```python
from build123d import *

# Parameters (mm, degrees)
F0_R     = 10.978044
F0_W     = 4.940685
F0_H     = 7.991237
F0_R_2   = 1.481086
F0_W_2   = 4.940115
F0_H_2   = 7.966079
F0_W_3   = 5.002896
F0_H_3   = 8.001204
F0_R_3   = 1.470755
F0_W_4   = 4.997425
F0_H_4   = 7.974718
F1_DEPTH = 5.0038


with BuildPart() as f1:
    # F0 (on Front) → F1 (new body)
    with BuildSketch(Plane.XZ):
        Polygon((29.282646, 29.627208), (-30.758047, 29.627208), (-30.758047, -12.548319), (-22.847719, -12.548319), (-22.847719, -63.122556), (21.501994, -63.122556), (21.501994, -12.548319), (29.282646, -12.548319), align=None)
        with BuildLine():
            ThreePointArc((-15.586378, -40.243281), (-17.742358, -40.254847), (-17.64737, -38.100929))
            Line((-17.64737, -38.100929), (-14.625554, -35.052073))
            ThreePointArc((-14.625554, -35.052073), (-12.57034, -35.03634), (-12.541453, -37.091411))
            Line((-12.541453, -37.091411), (-15.586378, -40.243281))
        make_face(mode=Mode.SUBTRACT)
        with BuildLine():
            ThreePointArc((16.426139, -38.233279), (16.534977, -40.292482), (14.478289, -40.441467))
            Line((14.478289, -40.441467), (11.236794, -37.068415))
            ThreePointArc((11.236794, -37.068415), (11.464462, -35.022049), (13.520983, -35.12287))
            ThreePointArc((13.520983, -35.12287), (13.537568, -35.140344), (13.55387, -35.158081))
            Line((13.55387, -35.158081), (16.426139, -38.233279))
        make_face(mode=Mode.SUBTRACT)
        with Locations((-0.654383, -23.181881)):
            Circle(F0_R, mode=Mode.SUBTRACT)
        with Locations((-25.189546, -3.442893)):
            Rectangle(F0_W, F0_H, mode=Mode.SUBTRACT)
        with BuildLine():
            ThreePointArc((-17.563489, -8.410167), (-17.594804, -6.240676), (-15.426944, -6.330432))
            Line((-15.426944, -6.330432), (-12.764063, -8.947979))
            ThreePointArc((-12.764063, -8.947979), (-12.531586, -11.12918), (-14.723433, -11.21573))
            Line((-14.723433, -11.21573), (-17.563489, -8.410167))
        make_face(mode=Mode.SUBTRACT)
        with Locations((-25.166028, 8.524365)):
            Circle(F0_R_2, mode=Mode.SUBTRACT)
        with Locations((-25.189262, 20.554467)):
            Rectangle(F0_W_2, F0_H_2, mode=Mode.SUBTRACT)
        with BuildLine():
            ThreePointArc((14.199827, -6.306034), (16.317638, -6.34597), (16.353841, -8.463848))
            Line((16.353841, -8.463848), (13.079717, -11.405483))
            ThreePointArc((13.079717, -11.405483), (10.953875, -11.342186), (11.064754, -9.218293))
            Line((11.064754, -9.218293), (14.199827, -6.306034))
        make_face(mode=Mode.SUBTRACT)
        with Locations((23.799085, -3.43791)):
            Rectangle(F0_W_3, F0_H_3, mode=Mode.SUBTRACT)
        with Locations((23.838598, 8.52569)):
            Circle(F0_R_3, mode=Mode.SUBTRACT)
        with Locations((23.80182, 20.558786)):
            Rectangle(F0_W_4, F0_H_4, mode=Mode.SUBTRACT)
    extrude(amount=F1_DEPTH)


solid = f1.part
```
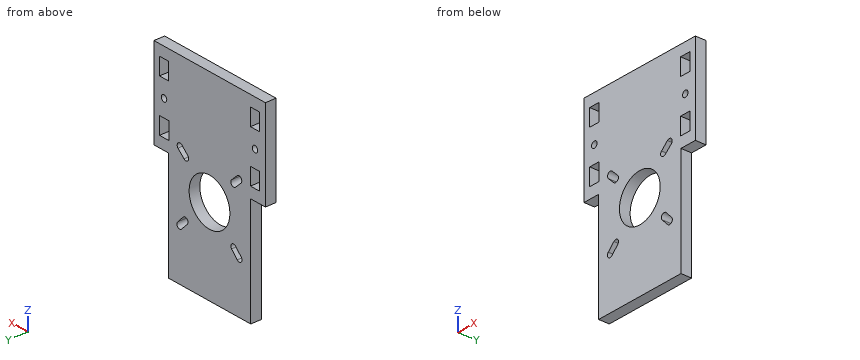
Here's how the part is built. I have some questions about the finished solid (model axes, mm). Give positions to 0.01 mm unless a question says otherwise; leave off trailing zeros. Order: outer loops, then holes, each group sorted by start corner. A loop starts at its lowest first (then second) coordinate and runs counter-clockwise, first axis right, second up. Notation, with made-up numbers: (7.5, 79) - (54.5, 79) arc R17 ccw to (54.5, 83) - close; hole circle Ø5 at (57.5, 8.5). An arc over 180 degrees is marked (long way). Answer as a JSON object with one key per item and string values. Group by question number.
Item 1: If we section it at C-C on x = -7.5: Please give me the cut outline in (y, z), and give its area (3 significant figures).
Item 2: If we section it at D-D on y = -3.5: Give the number of separate pieces and of enclosed holes in the cut face, and give its area (3 significant figures).
Item 3: If we section it at B-B on z = -28: Please give me the cut outline in (x, y), and give its area (3 significant figures).
Item 4: For P1, Ø1.5, axis at x = -25.5, y = -3, coming from the -Z side; P2, Ø1.5, axis at y = -3.5, z = -29, coming from the -X side; P3, Ø2.5, axis at y = -2.5, z = -47, coming from the +X side, each with a flat end and sliding along its axis, tell me the tip position at first contact or that it passes through.
Item 5: If we section it at A-A on z = -0.5: Please give me the cut outline in (x, y), and give its area (3 significant figures).
Item 6: Please list where these lines run through material, in increasing order: probe 1 along X at (y, z) = (-1.7, 21.5); probe 2 along Z at (x, y) = (24, -2.2); probe 3 along Z at (x, y) = (-26, -2.85).
Result set:
{
 "1": {"outline": "(-5, -63.12) - (0, -63.12) - (0, -31.76) - (-5, -31.76) - close; (-5, -14.6) - (0, -14.6) - (0, 29.63) - (-5, 29.63) - close", "area": "378 mm²"},
 "2": {"separate pieces": "1", "enclosed holes": "11", "area": "4,150 mm²"},
 "3": {"outline": "(-22.85, -5) - (-10.52, -5) - (-10.52, 0) - (-22.85, 0) - close; (9.21, -5) - (21.5, -5) - (21.5, 0) - (9.21, 0) - close", "area": "123 mm²"},
 "4": {"P1": "z = -12.55", "P2": "x = -22.85", "P3": "x = 21.5"},
 "5": {"outline": "(-30.76, -5) - (-27.66, -5) - (-27.66, 0) - (-30.76, 0) - close; (-22.72, -5) - (21.3, -5) - (21.3, 0) - (-22.72, 0) - close; (26.3, -5) - (29.28, -5) - (29.28, 0) - (26.3, 0) - close", "area": "251 mm²"},
 "6": {"probe 1": "-30.76 to -27.66, -22.72 to 21.3, 26.3 to 29.28", "probe 2": "-12.55 to -7.44, 0.56 to 7.06, 9.99 to 16.57, 24.55 to 29.63", "probe 3": "-12.55 to -7.44, 0.55 to 7.3, 9.75 to 16.57, 24.54 to 29.63"}
}
